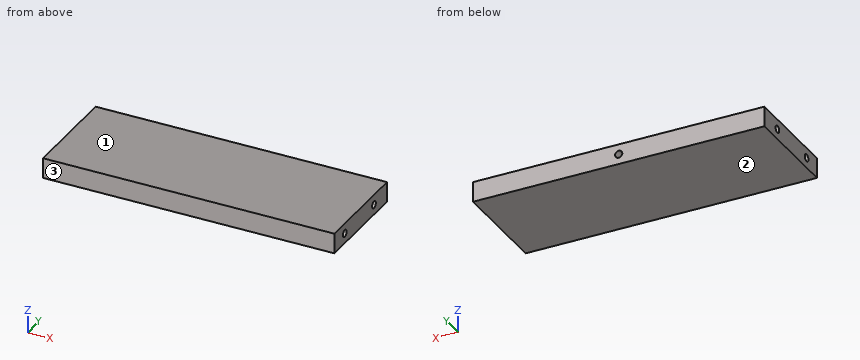
```python
from build123d import *

# Parameters (mm, degrees)
SKETCH1_W           = 91.44
SKETCH1_H           = 6.35
BOSS_EXTRUDE1_DEPTH = 32.131
SKETCH2_R           = 1.1303
CUT_EXTRUDE1_DEPTH  = 12.7
SKETCH3_R           = 1.1303
CUT_EXTRUDE2_DEPTH  = 12.7


with BuildPart() as part:
    # Sketch1 → Boss-Extrude1 (new body)
    with BuildSketch(Plane(origin=(0, 0, 0), x_dir=(1, 0, 0), z_dir=(0, 1, 0))):
        with Locations((-45.72, -3.175)):
            Rectangle(SKETCH1_W, SKETCH1_H)
    extrude(amount=BOSS_EXTRUDE1_DEPTH)

    # Sketch2 → Cut-Extrude1 (cut)
    with BuildSketch(Plane(origin=(0, 0, 0), x_dir=(0, 0, -1), z_dir=(1, 0, 0))):
        with Locations((-3.175, 24.1808)):
            Circle(SKETCH2_R)
        with Locations((-3.175, 6.35)):
            Circle(SKETCH2_R)
    cut_extrude1 = extrude(amount=-CUT_EXTRUDE1_DEPTH, mode=Mode.SUBTRACT)

    # Mirror2: Cut-Extrude1 across plane
    add(cut_extrude1.mirror(Plane(origin=(-45.72, 0, 0), x_dir=(0, 0, 1), z_dir=(1, 0, 0))), mode=Mode.SUBTRACT)

    # Sketch3 → Cut-Extrude2 (cut)
    with BuildSketch(Plane(origin=(0, 32.131, 0), x_dir=(1, 0, 0), z_dir=(0, 1, 0))):
        with Locations((-45.72, -3.175)):
            Circle(SKETCH3_R)
    extrude(amount=-CUT_EXTRUDE2_DEPTH, mode=Mode.SUBTRACT)


solid = part.part
```
Source: CAD feature listing. Evaluate the final solid. Frame: model axes, mm. Face numbers are marked on the shaded views. Round coordinates to 2 decimals unless told otherwise and drop trailing zeros. Order: outer loops, then holes, each group sorted by start corner. A loop starts at its lowest first (then second) coordinate and runs counter-clockwise, first axis right, second up. Notation, with made-up numbers: (38, 37) -> (42, 37) arc R33 cw to (42, 72) -> close; hole circle Ø1 at (29, 81.25). An arc over 180 degrees is marked (long way). One line per item, written item: value. Start each with the question number.
Q1. Pin query (flat end, axial travel): pin 1 (1.1 mm diameter, centred on y = 6, z = 3, fed in from +X); pin 2 (1.1 mm diameter, centred on x = -45.5, z = 3.5, fed in from +Y); pin 3 (1.1 mm diameter, centred on y = 6.5, z = 3.5, fed in from -X). Return the tip coordinate at first contact, or that it passes through.
Q2. Draft query along Z for the marked faces 1, 2 and 3. Return one class per face: pulls with the +Z half, pulls with the -Z half, needs draft (parallel to the pull), parting line crosses it, or undercut.
Q3. Section query C-C (x = -6). Return the cut outline in (y, z) (3 decimals).
Q4. Section query A-A (x = -45.72). Return the cut outline in (y, z), plus the area to 3 significant figures.
Q5. Material intervals for probe 1 along Y at (x, z) = (-84.5, 4); probe 2 along X at (y, z) = (25.5, 3); probe 3 along Y at (x, z) = (-80, 2.75), sorted ascending.
Q6. Section query B-B (y = 6.35). Return the cut outline in (x, z).
Findings below:
1. pin 1: x = -12.7
1. pin 2: y = 19.43
1. pin 3: x = -78.74
2. face 1: pulls with the +Z half
2. face 2: pulls with the -Z half
2. face 3: needs draft
3. outline: (0, 0) -> (32.131, 0) -> (32.131, 6.35) -> (0, 6.35) -> close; hole circle Ø2.261 at (6.35, 3.175); hole circle Ø2.261 at (24.181, 3.175)
4. outline: (0, 0) -> (32.13, 0) -> (32.13, 2.04) -> (19.43, 2.04) -> (19.43, 4.31) -> (32.13, 4.31) -> (32.13, 6.35) -> (0, 6.35) -> close
4. area: 175 mm²
5. probe 1: 0 to 5.58, 7.12 to 23.41, 24.95 to 32.13
5. probe 2: -91.44 to -46.84, -44.6 to 0
5. probe 3: 0 to 5.3, 7.4 to 23.13, 25.23 to 32.13
6. outline: (-91.44, 0) -> (0, 0) -> (0, 2.04) -> (-12.7, 2.04) -> (-12.7, 4.31) -> (0, 4.31) -> (0, 6.35) -> (-91.44, 6.35) -> (-91.44, 4.31) -> (-78.74, 4.31) -> (-78.74, 2.04) -> (-91.44, 2.04) -> close
